The listing builds one solid part. Answer for the finished solid, in the listing's coordinates (mm). A direction names the side the tool comes from. Give positions to 0.01 mm unless a question says otherwise; leave off trailing zeros. Loops run counter-clockwise (first coordinate to the right, second up) from the corner with the lowest first, then second, coordinate; pieces in that order, holes last.
Item 1: Each of these flat-tipped pins is pushed along its axis until it touches: pin 1 Ø0.9 at (y, z) = (-81, 1.5) entering from +X; pin 2 Ø0.9 at (y, z) = (-81.5, 1.5) entering from -X; pin 3 Ø0.5 at (x, y) = (-174, -42) entering from -Z. Where does it stop, or does it pass through?
Item 2: Section A-A, the plane y = -34 is taken. Give the vertices of the cut face in (x, z), and give its area (4 significant figures).
Item 3: Section C-C, the plane y = -15 is taken. Give the vertices of the cut face in (x, z).
Item 4: Section D-D, the plane x = -138 is taken. Give the vertices of the cut face in (y, z).
Item 5: A tool of negligible diameter and unlimited length cuts with its end or side. For faces 1 (the face through (-44, -80, 1)), 2 (the face through (-106.75, -81, 2)), 3 (the face through (-9, -40, 1)), from which of +Z, -Z, +X, -X, +Y, -Y can it reach the whole face along a straight path? Write none if from no direction.
Item 6: Section B-B, the plane z = 0.6 is taken. Give the vertices of the cut face in (x, y), and give its area (3 significant figures).
Item 7: Consider line 1 along X through (y, z) = (-25, 0.2); line 2 along X through (y, z) = (-33.5, 1.35); line 3 along X through (y, z) = (-28, 1.9). Determine where each line is inside the solid, lowest interval first.
from build123d import *

# Parameters (mm, degrees)
ESQUISSE2_W             = 175
ESQUISSE2_H             = 80
BOSS_EXTRU_2_DEPTH      = 3
ENL_V_MAT_EXTRU_1_REACH = 194.442
ESQUISSE3_W             = 3
ESQUISSE3_H             = 20
ENL_V_MAT_EXTRU_2_REACH = 194.442
ESQUISSE4_W             = 1
ESQUISSE4_H             = 1.5
ESQUISSE5_W             = 20
ESQUISSE5_H             = 3
BOSS_EXTRU_3_DEPTH      = 3
ESQUISSE6_W             = 4
ESQUISSE6_H             = 20
ENL_V_MAT_EXTRU_3_DEPTH = 10


with BuildPart() as part:
    # Esquisse2 → Boss.-Extru.2 (new body)
    with BuildSketch(Plane.XY):
        with Locations((-87.5, -40)):
            Rectangle(ESQUISSE2_W, ESQUISSE2_H)
    extrude(amount=BOSS_EXTRU_2_DEPTH)

    # Esquisse3 → Enlèv. mat.-Extru.1 (cut, up to next)
    with BuildSketch(Plane.XY.offset(3), mode=Mode.PRIVATE) as enl_v_mat_extru_1_sk1:
        with Locations((-51.5, -60)):
            Rectangle(ESQUISSE3_W, ESQUISSE3_H)
    enl_v_mat_extru_1_tool1 = extrude(enl_v_mat_extru_1_sk1.sketch, amount=-ENL_V_MAT_EXTRU_1_REACH, mode=Mode.PRIVATE) & part.part
    # Esquisse3 → Enlèv. mat.-Extru.1 (cut, up to next)
    with BuildSketch(Plane.XY.offset(3), mode=Mode.PRIVATE) as enl_v_mat_extru_1_sk2:
        with Locations((-51.5, -20)):
            Rectangle(ESQUISSE3_W, ESQUISSE3_H)
    enl_v_mat_extru_1_tool2 = extrude(enl_v_mat_extru_1_sk2.sketch, amount=-ENL_V_MAT_EXTRU_1_REACH, mode=Mode.PRIVATE) & part.part
    add(enl_v_mat_extru_1_tool1.solids().sort_by_distance((-51.5, -60, 3))[0], mode=Mode.SUBTRACT)
    add(enl_v_mat_extru_1_tool2.solids().sort_by_distance((-51.5, -20, 3))[0], mode=Mode.SUBTRACT)

    # Esquisse4 → Enlèv. mat.-Extru.2 (cut, up to next)
    with BuildSketch(Plane(origin=(0, 0, 0), x_dir=(1, 0, 0), z_dir=(0, 1, 0)), mode=Mode.PRIVATE) as enl_v_mat_extru_2_sk1:
        with Locations((-174, -0.75)):
            Rectangle(ESQUISSE4_W, ESQUISSE4_H)
    enl_v_mat_extru_2_tool1 = extrude(enl_v_mat_extru_2_sk1.sketch, amount=-ENL_V_MAT_EXTRU_2_REACH, mode=Mode.PRIVATE) & part.part
    add(enl_v_mat_extru_2_tool1.solids().sort_by_distance((-174, 0, 0.75))[0], mode=Mode.SUBTRACT)

    # Esquisse5 → Boss.-Extru.3 (add)
    with BuildSketch(Plane(origin=(0, -80, 0), x_dir=(-1, 0, 0), z_dir=(0, -1, 0))):
        with Locations((96.75, -1.5)):
            Rectangle(ESQUISSE5_W, ESQUISSE5_H)
    extrude(amount=BOSS_EXTRU_3_DEPTH)

    # Esquisse6 → Enlèv. mat.-Extru.3 (cut)
    with BuildSketch(Plane(origin=(0, 0, 0), x_dir=(-1, 0, 0), z_dir=(0, 0, -1))):
        with Locations((7, -40)):
            Rectangle(ESQUISSE6_W, ESQUISSE6_H)
    extrude(amount=-ENL_V_MAT_EXTRU_3_DEPTH, mode=Mode.SUBTRACT)


solid = part.part
Worked answers:
1. pin 1: stops at x = -86.75
1. pin 2: stops at x = -106.75
1. pin 3: stops at z = 1.5
2. outline: (-175, 0) - (-174.5, 0) - (-174.5, 1.5) - (-173.5, 1.5) - (-173.5, 0) - (-9, 0) - (-9, 3) - (-175, 3) - close; (-5, 0) - (0, 0) - (0, 3) - (-5, 3) - close
2. area: 511.5 mm2
3. outline: (-175, 0) - (-174.5, 0) - (-174.5, 1.5) - (-173.5, 1.5) - (-173.5, 0) - (-53, 0) - (-53, 3) - (-175, 3) - close; (-50, 0) - (0, 0) - (0, 3) - (-50, 3) - close
4. outline: (-80, 0) - (0, 0) - (0, 3) - (-80, 3) - close
5. face 1: +Z, -Z, +X, -Y
5. face 2: +Z, -Z, -X, -Y
5. face 3: +Z, -Z
6. outline: (-175, -80) - (-174.5, -80) - (-174.5, 0) - (-175, 0) - close; (-173.5, -80) - (-106.75, -80) - (-106.75, -83) - (-86.75, -83) - (-86.75, -80) - (0, -80) - (0, 0) - (-173.5, 0) - close; hole (-53, -70) - (-50, -70) - (-50, -50) - (-53, -50) - close; hole (-53, -30) - (-50, -30) - (-50, -10) - (-53, -10) - close; hole (-9, -50) - (-5, -50) - (-5, -30) - (-9, -30) - close
6. area: 13,800 mm2
7. line 1: x = -175 to -174.5, -173.5 to -53, -50 to 0
7. line 2: x = -175 to -174.5, -173.5 to -9, -5 to 0
7. line 3: x = -175 to -53, -50 to 0
